```python
from build123d import *

# Parameters (mm, degrees)
EXTRUDE_SKETCH_1_R = 12.16
EXTRUDE_1_DEPTH    = 2.16
EXTRUDE_START      = 2.16
EXTRUDE_2_DEPTH    = 7.8
EXTRUDE_START_2    = -130
EXTRUDE_SKETCH_3_R = 6
EXTRUDE_3_DEPTH    = 130.01


with BuildPart() as part:
    # Extrude sketch 1 → Extrude 1 (new body)
    with BuildSketch(Plane.XY):
        Circle(EXTRUDE_SKETCH_1_R)
    extrude(amount=EXTRUDE_1_DEPTH)


with BuildPart() as body_2:
    # Extrude sketch 2 → Extrude 2 (new body)
    with BuildSketch(Plane.XY.offset(EXTRUDE_START)):
        Polygon((9, 5.196152423), (0, 10.392304845), (-9, 5.196152423), (-9, -5.196152423), (0, -10.392304845), (9, -5.196152423), align=None)
    extrude(amount=EXTRUDE_2_DEPTH)


with BuildPart() as body_3:
    # Extrude sketch 3 → Extrude 3 (new body)
    with BuildSketch(Plane.XY.offset(EXTRUDE_START_2)):
        Circle(EXTRUDE_SKETCH_3_R)
    extrude(amount=EXTRUDE_3_DEPTH)

    # Combine (weld / assembly of features): union body 2, part
    add(body_2.part)
    add(part.part)


solid = body_3.part
```
Read the model definition and answer for the solid it produces. Units are mm, in the model's axes. A direction names the side the tool comes from. Give positions to 0.01 mm unless a question says otherwise; leave off trailing zeros. Write each loop counter-clockwise with the first axis right and the second up, starting at its lowest first coordinate (ties: lowest second). Pieces come first, ordered by that corner, then holes. Notation, with made-up numbers: (85, -32.75) -> (91, -32.75) arc R17 cw to (91, -7.75) -> close; hole circle Ø8 at (-10.5, -8). An arc over 180 degrees is marked (long way). Answer as a JSON object with one key per item and string values.
1) Flat-ended cylindrical pins translate along their axes: pin 1 Ø1.5 at (y, z) = (-2.5, -57.5) entering from +X; pin 2 Ø3 at (x, y) = (-6, -6.5) entering from -Z; pin 3 Ø12 at (y, z) = (6.5, -8.5) entering from -X. Find the tip coordinate at first contact, or state that the pin passes through.
Findings below:
{"pin 1": "stops at x = 5.74", "pin 2": "stops at z = 0", "pin 3": "stops at x = -5.98"}
2) A tool of negligible diameter and unlimited length cuts with its end or side. For faces 1 (the flat face through (-7.3, 6.4, 2.16)), 2 (the flat face through (4.44, -7.83, 6.01)), 3 (the flat face through (-4.44, 7.83, 6.01)), 4 (the flat face through (9, 0, 6)), from which of +Z, -Z, +X, -X, +Y, -Y can it reach the whole face along a straight path? Write none if from no direction.
Findings below:
{"face 1": "+Z", "face 2": "+Z, +X, -Y", "face 3": "+Z, -X, +Y", "face 4": "+Z, +X, +Y, -Y"}
3) For a pull along Y with two mould halves and no side action, classify faces 5 (the flat face through (-4.56, -7.76, 6.01)), 6 (the flat face through (0, 0, 9.96)), 7 (the cylindrical face through (11.6, 3.65, 1.06)), 8 (the flat face through (4.56, 7.76, 6.01)) as pulls with the +Y half, pulls with the -Y half, needs draft (parallel to the pull), parting line crosses it, or undercut.
Findings below:
{"face 5": "pulls with the -Y half", "face 6": "needs draft", "face 7": "parting line crosses it", "face 8": "pulls with the +Y half"}
4) Section A-A on y = 0 is taken. Write down the section's boundary in (x, z), then the cut area to 3 significant figures.
Findings below:
{"outline": "(-12.16, 0) -> (-6, 0) -> (-6, -130) -> (6, -130) -> (6, 0) -> (12.16, 0) -> (12.16, 2.16) -> (9, 2.16) -> (9, 9.96) -> (-9, 9.96) -> (-9, 2.16) -> (-12.16, 2.16) -> close", "area": "1,750 mm^2"}
5) Straight lines are drawn through the part: probe 1 along Z at (x, y) = (-8.5, 6.25); probe 2 along Z at (x, y) = (-4.25, -4.5); probe 3 along Y at (x, z) = (-0.5, -102). For each, find the intervals that lie inside material, in ascending order. Write a range as from..to.
Findings below:
{"probe 1": "z = 0..2.16", "probe 2": "z = 0..9.96", "probe 3": "y = -5.98..5.98"}
6) Section D-D on x = 10.5 is taken. Write down the section's boundary in (y, z), then the cut area to 3 significant figures.
Findings below:
{"outline": "(-6.13, 0) -> (6.13, 0) -> (6.13, 2.16) -> (-6.13, 2.16) -> close", "area": "26.5 mm^2"}
7) Section C-C on z = -6.5 is taken. Write down the section's boundary in (x, y), then the cut area to 3 significant figures.
Findings below:
{"outline": "circle Ø12 at (0, 0)", "area": "113 mm^2"}
8) Section B-B on x = -2 is taken. Write down the section's boundary in (y, z).
Findings below:
{"outline": "(-11.99, 0) -> (-5.66, 0) -> (-5.66, -130) -> (5.66, -130) -> (5.66, 0) -> (11.99, 0) -> (11.99, 2.16) -> (9.24, 2.16) -> (9.24, 9.96) -> (-9.24, 9.96) -> (-9.24, 2.16) -> (-11.99, 2.16) -> close"}
